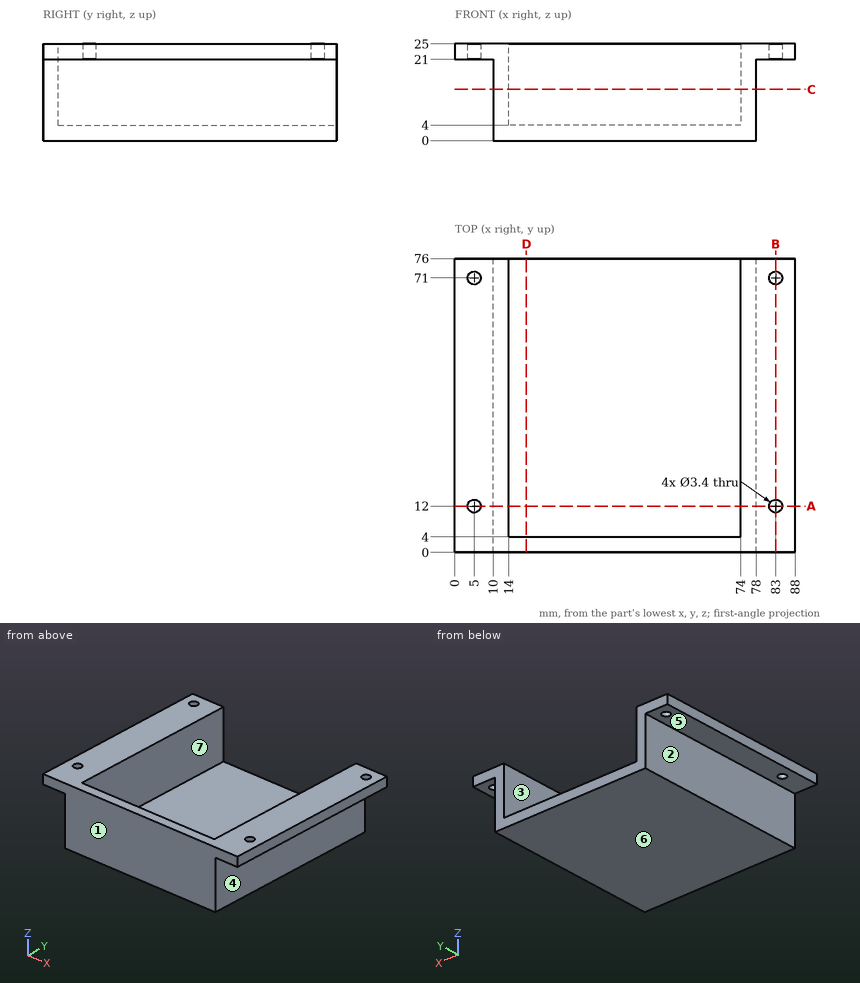
Input: dimensioned drawing with shaded views. Units: mm. Origin: part minimum x, y, z. A direction names the side the tool comes from. Coordinates: 2 decimals unless noted, no trailing zeros. Order: outer loops, then holes, each group sorted by start corner. A loop starts at its lowest first (then second) coordinate and runs counter-clockwise, first axis right, second up.
(1) Section query D-D (x = 18.5). Return the cut outline in (y, z), plus the area to 3 significant figures.
(2) Access query for the marked faces 4, 5, 6 and 7. Directions: +Z, -Z, +X, -X, +Y, -Y. A direction counts if a zero-diameter tool reaches every point of the face in a straight line with its end or side. Return the directions, or none.
(3) Material intervals for probe 1 along Y at (x, z) = (83, 23); probe 2 along X at (y, z) = (71, 22.15); probe 3 along X at (y, z) = (33, 5), sorted ascending.
(4) Section query B-B (x = 83). Return the cut outline in (y, z).
(5) Section query A-A (y = 12). Return the cut outline in (x, z), plus the area to 3 significant figures.
(6) Section query C-C (z = 13.25). Return the cut outline in (x, y), plus the area to 3 significant figures.
(7) First-contact query: pin 1 (6.5 mm diameter, centred on y = 46.5, z = 10.5, fed in from +X); pin 2 (10.5 mm diameter, centred on y = 33.5, z = 15, fed in from -X); pin 3 (1 mm diameter, centred on x = 68.5, z = 17.5, fed in from -Y); pin 4 (8 mm diameter, centred on x = 18.5, y = 45.5, fed in from +Z). Flat tips, straight axial feed; report the tip coordinate or a pass-through.
(8) Draft query along X for the marked faces 1, 2 and 3. Return one class per face: pulls with the +X half, pulls with the -X half, needs draft (parallel to the pull), parting line crosses it, or undercut.
Solution:
1. outline: (0, 0) - (76, 0) - (76, 4) - (4, 4) - (4, 25) - (0, 25) - close
1. area: 388 mm2
2. face 4: -Z, +X, +Y, -Y
2. face 5: -Z, -X, +Y, -Y
2. face 6: -Z, +X, -X, +Y, -Y
2. face 7: +Z, +Y
3. probe 1: y = 0 to 10.3, 13.7 to 69.3, 72.7 to 76
3. probe 2: x = 0 to 3.3, 6.7 to 14, 74 to 81.3, 84.7 to 88
3. probe 3: x = 10 to 14, 74 to 78
4. outline: (0, 21) - (10.3, 21) - (10.3, 25) - (0, 25) - close; (13.7, 21) - (69.3, 21) - (69.3, 25) - (13.7, 25) - close; (72.7, 21) - (76, 21) - (76, 25) - (72.7, 25) - close
5. outline: (0, 21) - (3.3, 21) - (3.3, 25) - (0, 25) - close; (6.7, 21) - (10, 21) - (10, 0) - (78, 0) - (78, 21) - (81.3, 21) - (81.3, 25) - (74, 25) - (74, 4) - (14, 4) - (14, 25) - (6.7, 25) - close; (84.7, 21) - (88, 21) - (88, 25) - (84.7, 25) - close
5. area: 493 mm2
6. outline: (10, 0) - (78, 0) - (78, 76) - (74, 76) - (74, 4) - (14, 4) - (14, 76) - (10, 76) - close
6. area: 848 mm2
7. pin 1: stops at x = 78
7. pin 2: stops at x = 10
7. pin 3: stops at y = 0
7. pin 4: stops at z = 4
8. face 1: needs draft
8. face 2: pulls with the -X half
8. face 3: undercut
